Autodesk Inventor part; units mm, degrees
ref_plane "Work Plane1" through (0, 45, 27) normal (1, 0, 0) x (0, 0, -1)
ref_plane "Work Plane2" through (0, 45, -81) normal (-1, 0, 0) x (0, 0, 1)
ref_plane "YZ Plane" through (0, 0, 0) normal (1, 0, 0) x (0, 1, 0)
sketch "Sketch1" plane through (0, 0, 0) normal (0, 0, 1) x (1, 0, 0)
  line L0 (-31, -31) -> (31, -31)
  line L1 (31, -31) -> (31, 31)
  line L2 (31, 31) -> (-31, 31)
  line L3 (-31, 31) -> (-31, -31)
  line L4 (-31, -31) -> (31, 31) construction
  line L5 (31, -31) -> (-31, 31) construction
  line L6 (-33, 33) -> (33, 33)
  line L7 (33, 33) -> (33, -33)
  line L8 (33, -33) -> (-33, -33)
  line L9 (-33, -33) -> (-33, 33)
  point P0 (0, 0)
  dimension "d0" = 62
  dimension "d1" = 62
  dimension "d2" = 2
extrude "Extrusion1" add sketch "Sketch1" along normal blind 2 contours L3 L2 L1 L0 | L6 L7 L8 L9
extrude "Extrusion2" add sketch "Sketch1" against normal blind 12
sketch "Sketch2" plane through (-33, 33, 2) normal (0, 1, 0) x (1, 0, 0)
  line L0 (13, 3) -> (53, 3)
  line L1 (53, 3) -> (53, 0)
  line L2 (53, 0) -> (13, 0)
  line L3 (13, 0) -> (13, 3)
  line L4 (0, 14) -> (0, 0)
  line L5 (0, 14) -> (66, 14)
  point P0 (33, 2)
  dimension "d7" = 40
  dimension "d8" = 3
  dimension "d9" = 13
  dimension "d10" = 11
extrude "Extrusion3" add sketch "Sketch2" along normal blind 12
sketch "Sketch3" plane through (20, 33, -1) normal (0, 0, -1) x (-1, 0, 0)
  line L0 (40, 12) -> (0, 12)
  line L1 (40, 0) -> (40, 12)
  line L2 (0, 12) -> (40, 12)
  line L3 (40, 12) -> (40, 9)
  line L4 (40, 9) -> (0, 9)
  line L5 (0, 9) -> (0, 12)
  point P0 (20, -33)
  dimension "d13" = 3
extrude "Extrusion4" add sketch "Sketch3" along normal blind 80
sketch "Sketch4" plane through (-20, 42, -1) normal (0, -1, 0) x (1, 0, 0)
  line L0 (30.5, -63) -> (9.5, -63)
  line L1 (9.5, -63) -> (9.5, -22)
  line L2 (9.5, -22) -> (30.5, -22)
  line L3 (30.5, -22) -> (30.5, -63)
  line L4 (40, 3) -> (40, -80)
  line L5 (0, 3) -> (40, 3)
  point P0 (20, 1)
  dimension "d16" = 21
  dimension "d17" = 41
  dimension "d18" = 9.5
  dimension "d19" = 25
extrude "Extrusion5" cut sketch "Sketch4" against normal blind 80
sketch "Sketch5" plane through (-20, 42, -1) normal (0, -1, 0) x (1, 0, 0)
  line L0 (30.5, -63) -> (9.5, -63)
  line L1 (30.5, -63) -> (9.5, -63)
  line L2 (9.5, -63) -> (9.5, -70)
  line L3 (9.5, -70) -> (30.5, -70)
  line L4 (30.5, -70) -> (30.5, -63)
  circle A0 centre (15, -66.75) radius 2.25
  line L5 (30.5, -22) -> (30.5, -63)
  line L6 (30.5, -22) -> (9.5, -22)
  line L7 (9.5, -22) -> (9.5, -15)
  line L8 (9.5, -15) -> (30.5, -15)
  line L9 (30.5, -15) -> (30.5, -22)
  circle A1 centre (25, -18.5) radius 2.25
  point P0 (20, 1)
  point P1 (14.9217, -69.81)
  point P2 (13.9783, -69.81)
  point P3 (25.0283, -15.19)
  point P4 (25.9717, -15.19)
  dimension "d22" = 7
  dimension "d23" = 4.5
  dimension "d24" = 3.75
  dimension "d25" = 5.5
  dimension "d26" = 7
  dimension "d27" = 4.5
  dimension "d28" = 5.5
  dimension "d29" = 3.5
extrude "Extrusion6" cut sketch "Sketch5" against normal blind 80 contours A0 | A1
sketch "Sketch6" plane through (-33, -33, 2) normal (0, -1, 0) x (1, 0, 0)
  line L0 (0, -14) -> (0, 0)
  line L1 (66, -14) -> (66, 0)
  line L2 (0, 0) -> (66, 0)
  line L3 (66, 0) -> (66, -14)
  line L4 (66, -14) -> (0, -14)
  line L5 (0, -14) -> (0, 0)
  point P0 (33, -2)
  point P1 (66, 0)
extrude "Extrusion7" cut sketch "Sketch6" against normal up to surface (75 mm away)
sketch "Sketch7" plane through (0, 0, 2) normal (0, 0, 1) x (1, 0, 0)
  line L0 (-20, 42) -> (-20, 45)
  line L1 (20, 42) -> (20, 45)
  line L2 (-20, 45) -> (20, 45)
  line L3 (20, 45) -> (20, 42)
  line L4 (20, 42) -> (-20, 42)
  line L5 (-20, 42) -> (-20, 45)
  point P0 (0, 0)
extrude "Extrusion8" add sketch "Sketch7" along normal blind 25
sketch "Sketch8" plane through (-20, 42, -81) normal (0, -1, 0) x (1, 0, 0)
  line L0 (0, 108) -> (0, 0)
  line L1 (40, 0) -> (40, 108)
  line L2 (0, 108) -> (40, 108)
  line L3 (40, 108) -> (40, 105)
  line L4 (40, 105) -> (0, 105)
  line L5 (0, 105) -> (0, 108)
  point P0 (20, 81)
  dimension "d36" = 3
extrude "Extrusion9" add sketch "Sketch8" along normal blind 100
sketch "Sketch9" plane through (20, 42, 24) normal (0, 0, -1) x (-1, 0, 0)
  circle A0 centre (20, -90) radius 2
  circle A1 centre (8, -50) radius 2
  circle A2 centre (32, -20) radius 2
  line L0 (40, 0) -> (40, -100)
  line L1 (0, 0) -> (0, -100)
  line L2 (40, -100) -> (0, -100)
  line L3 (0, 0) -> (40, 0)
  point P0 (20, -42)
  dimension "d39" = 4
  dimension "d40" = 4
  dimension "d41" = 4
  dimension "d42" = 8
  dimension "d43" = 8
  dimension "d44" = 20
  dimension "d45" = 10
  dimension "d46" = 50
  dimension "d47" = 20
extrude "Extrusion10" cut sketch "Sketch9" against normal blind 10 contours A0 | A1 | A2
ref_plane "Work Plane1" through (0, 45, 27) normal (1, 0, 0) x (0, 0, -1)
sketch "Sketch11" plane through (20, 45, 27) normal (1, 0, 0) x (0, 0, -1)
  line L0 (3, -3) -> (3, -103)
  line L1 (3, -3) -> (103, -3)
  line L2 (103, -3) -> (103, -19)
  line L3 (103, -19) -> (3, -19)
  line L4 (3, -19) -> (3, -3)
  line L5 (103, -3) -> (3, -19)
  point P0 (27, -45)
  point P1 (3, -19)
  dimension "d55" = 100
  dimension "d56" = 16
extrude "Extrusion12" add sketch "Sketch11" against normal blind 4 contours L1 L5 L0
ref_plane "Work Plane2" through (0, 45, -81) normal (-1, 0, 0) x (0, 0, 1)
mirror "Mirror1" about plane through (0, 45, -81) normal (-1, 0, 0) of "Extrusion12"
properties part number "pan_base_holder_first"
Read the model definition and answer for the solid it produces. Units are mm, in the model's axes. A direction names the side the tool comes from. Give positions to 0.01 mm unless a question says otherwise; leave off trailing zeros. Write each loop counter-clockwise with the first axis right and the second up, starting at its lowest first coordinate (ties: lowest second). Pieces come first, ordered by that corner, then holes. Notation, with made-up numbers: (44, 40) - (102, 40) arc R4 ccw to (102, 45) - close; hole circle Ø8 at (77, 64). An arc over 180 degrees is marked (long way). Answer in a Markdown table with one row per item. Add a question column.
Item 1: Determine the mould class of faces 1 (the face through (-0.923, -49.774, 25.479)), 2 (the face through (0, 42, -18)), 3 (the face through (13.474, -6.648, 25.479)), 4 (the face through (0, 44, -81)) for opening direction Y: pulls with the +Y half, pulls with the -Y half, needs draft (parallel to the pull), parting line crosses it, or undercut.
Item 2: Find the intervals of material crossed by L1, parallel to Y at x = -12, z = 26; L2, parallel to Y at x = 12, z = 25.65; L3, parallel to Z at x = -2, y = -42, in increasing order.
Item 3: Section C-C, the plane x = 12 is taken. Write down the section's boundary in (y, z).
Item 4: Section B-B, the plane z = -57 is taken. Write down the section's boundary in (x, y), and give its area (3 significant figures).
Item 5: Section D-D, the plane y = 22 is taken. Write down the section's boundary in (x, z).
Item 6: A tool of negligible diameter and unlimited length cuts with its end or side. For faces 5 (the face through (0, -58, 26)), 6 (the face through (0, 43, -64)), 7 (the face through (0, -7, 24)), from which of +Z, -Z, +X, -X, +Y, -Y can it reach the whole face along a straight path? Write none if from no direction.
Item 7: Section A-A, the plane x = 5 is taken. Write down the section's boundary in (y, z).
Item 8: Flat-ended cylindrical pins translate along their axes: P1, Ø1.5, axis at x = 12.5, z = -10.5, coming from the -Y side; P2, Ø12, axis at x = -2.5, y = -36, coming from the -Z side; P3, Ø5, axis at y = 33, z = -20, coming from the +X side. Find the tip coordinate at first contact, or state that the pin passes through.
Recorded:
| question | item | result |
|---|---|---|
| 1 | face 1 | undercut |
| 1 | face 2 | pulls with the -Y half |
| 1 | face 3 | undercut |
| 1 | face 4 | needs draft |
| 2 | L1 | y = -58 to 20, 24 to 45 |
| 2 | L2 | y = -58 to -10, -6 to 45 |
| 2 | L3 | z = 24 to 27 |
| 3 | outline | (-58, 24) - (-10, 24) - (-10, 27) - (-58, 27) - close; (-6, 24) - (42, 24) - (42, -81) - (45, -81) - (45, 27) - (-6, 27) - close |
| 4 | outline | (-20, 38.96) - (-16, 38.96) - (-16, 42) - (-10.5, 42) - (-10.5, 45) - (-20, 45) - close; (10.5, 42) - (16, 42) - (16, 38.96) - (20, 38.96) - (20, 45) - (10.5, 45) - close |
| 4 | area | 81.3 mm2 |
| 5 | outline | (-20, 24) - (-14, 24) - (-14, 27) - (-20, 27) - close; (-10, 24) - (20, 24) - (20, 27) - (-10, 27) - close |
| 6 | face 5 | +Z, -Z, +X, -X, -Y |
| 6 | face 6 | +Y, -Y |
| 6 | face 7 | -Z, -Y |
| 7 | outline | (-58, 24) - (42, 24) - (42, -17.25) - (45, -17.25) - (45, 27) - (-58, 27) - close; (42, -81) - (45, -81) - (45, -64) - (42, -64) - close; (42, -23) - (45, -23) - (45, -21.75) - (42, -21.75) - close |
| 8 | P1 | stops at y = 42 |
| 8 | P2 | stops at z = 24 |
| 8 | P3 | stops at x = 20 |
